```python
from build123d import *

# Parameters (mm, degrees)
SKETCH1_W           = 88.9
SKETCH1_H           = 50.8
BOSS_EXTRUDE1_DEPTH = 114.3
SKETCH2_OUTSIDE_W   = 121.59
SKETCH2_OUTSIDE_H   = 83.49
SKETCH2_OUTSIDE_W_2 = 50.8
SKETCH2_OUTSIDE_H_2 = 50.8
CUT_EXTRUDE1_DEPTH  = 101.6
SKETCH3_R           = 4.9609375
CUT_EXTRUDE2_DEPTH  = 114.769602707
SKETCH4_R           = 5.3578125
CUT_EXTRUDE3_DEPTH  = 41.275
SKETCH5_R           = 2.54
CUT_EXTRUDE4_DEPTH  = 2.54


with BuildPart() as part:
    # Sketch1 → Boss-Extrude1 (new body)
    with BuildSketch(Plane(origin=(0, 0, 0), x_dir=(1, 0, 0), z_dir=(0, 1, 0))):
        Rectangle(SKETCH1_W, SKETCH1_H)
    extrude(amount=BOSS_EXTRUDE1_DEPTH)

    # Sketch2 outside → Cut-Extrude1 (cut)
    with BuildSketch(Plane(origin=(0, 114.3, 0), x_dir=(1, 0, 0), z_dir=(0, 1, 0))):
        Rectangle(SKETCH2_OUTSIDE_W, SKETCH2_OUTSIDE_H)
        Rectangle(SKETCH2_OUTSIDE_W_2, SKETCH2_OUTSIDE_H_2, mode=Mode.SUBTRACT)
    extrude(amount=-CUT_EXTRUDE1_DEPTH, mode=Mode.SUBTRACT)

    # Sketch3 → Cut-Extrude2 (cut, through all)
    with BuildSketch(Plane(origin=(0, 12.7, 0), x_dir=(1, 0, 0), z_dir=(0, 1, 0))):
        with Locations(Location((-34.925, 15.875, 0), (0, 0, 270))):
            Circle(SKETCH3_R)
        with Locations(Location((-34.925, -15.875, 0), (0, 0, 270))):
            Circle(SKETCH3_R)
        with Locations(Location((34.925, -15.875, 0), (0, 0, 270))):
            Circle(SKETCH3_R)
        with Locations(Location((34.925, 15.875, 0), (0, 0, 270))):
            Circle(SKETCH3_R)
    extrude(amount=-CUT_EXTRUDE2_DEPTH, mode=Mode.SUBTRACT)

    # Sketch4 → Cut-Extrude3 (cut)
    with BuildSketch(Plane(origin=(0, 114.3, 0), x_dir=(1, 0, 0), z_dir=(0, 1, 0))):
        with Locations(Location((0, 0, 0), (0, 0, 270))):
            Circle(SKETCH4_R)
    extrude(amount=-CUT_EXTRUDE3_DEPTH, mode=Mode.SUBTRACT)

    # Sketch5 → Cut-Extrude4 (cut)
    with BuildSketch(Plane.XZ):
        with Locations(Location((0, 0, 0), (0, 0, 270))):
            Circle(SKETCH5_R)
    extrude(amount=-CUT_EXTRUDE4_DEPTH, mode=Mode.SUBTRACT)


solid = part.part
```
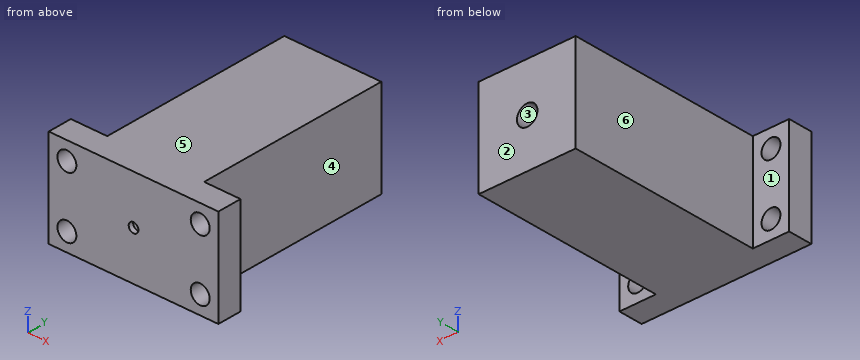
CAD build for the part. Positions are in the model's coordinates, mm. Face numbers are marked on the shaded views. A direction names the side the tool comes from. Round coordinates to 2 decimals unless told otherwise and drop trailing zeros. Write each loop counter-clockwise with the first axis right and the second up, starting at its lowest first coordinate (ties: lowest second). Pieces come first, ordered by that corner, then holes. Notation, with made-up numbers: (67.25, 37.25) - (85.25, 37.25) arc R10 ccw to (85.25, 55.25) - close; hole circle Ø2 at (18, 38.5). An arc over 180 degrees is marked (long way). Return JSON: item names as keys, results as strings. Group by question number.
Item 1: Flat gauge pins, fed straight in: pin 1 Ø8 at (y, z) = (82, -1.5) entering from -X; pin 2 Ø6 at (x, z) = (34.925, 15.875) entering from +Y; pin 3 Ø2.5 at (x, z) = (0.5, 1) entering from -Y; pin 4 Ø9.5 at (x, z) = (31, -9) entering from +Y. Where does each tip first touch, or does it go through?
Item 2: Band-saw the part on D-D on z = 0. List the corners of the cut face in (x, y) (3 decimals), plus the area to 3 significant figures.
Item 3: Band-saw the part on B-B on x = 0. List the corners of the cut face in (y, z) (3 decimals).
Item 4: Mould opens along X. For the marked faces 3, 4, 5 and 6 say: +X half, -X half, draft (parallel to the pull), parting line (faces both ways), or undercut.
Item 5: 3-axis set-ups, long thin cutter, end or side, ignore diameter. For the marked faces 1 and 2: which of +Z, -Z, +X, -X, +Y, -Y reach the whole face in a straight line?
Item 6: Band-saw the part on C-C on x = -32. List the corners of the cut face in (y, z), plus the area to 3 significant figures.
Item 7: Band-saw the part on A-A on z = 19.5. List the corners of the cut face in (x, y).
Item 8: Probe probe 1 along X at (y, z) = (98, 0); probe 2 along X at (y, z) = (7, -19.5); probe 3 along X at (y, z) = (76, 19). List the from-to ranges inside material, lowest first.
Resolved:
{
 "1": {"pin 1": "stops at x = -25.4", "pin 2": "passes through", "pin 3": "stops at y = 2.54", "pin 4": "stops at y = 12.7"},
 "2": {"outline": "(-44.45, 0) - (-2.54, 0) - (-2.54, 2.54) - (2.54, 2.54) - (2.54, 0) - (44.45, 0) - (44.45, 12.7) - (25.4, 12.7) - (25.4, 114.3) - (5.358, 114.3) - (5.358, 73.025) - (-5.358, 73.025) - (-5.358, 114.3) - (-25.4, 114.3) - (-25.4, 12.7) - (-44.45, 12.7) - close", "area": "5,840 mm²"},
 "3": {"outline": "(0, -25.4) - (114.3, -25.4) - (114.3, -5.358) - (73.025, -5.358) - (73.025, 5.358) - (114.3, 5.358) - (114.3, 25.4) - (0, 25.4) - (0, 2.54) - (2.54, 2.54) - (2.54, -2.54) - (0, -2.54) - close"},
 "4": {"face 3": "undercut", "face 4": "+X half", "face 5": "draft", "face 6": "-X half"},
 "5": {"face 1": "+Z, -Z, -X, +Y", "face 2": "+Z, -Z, +X, -X, +Y"},
 "6": {"outline": "(0, -25.4) - (12.7, -25.4) - (12.7, -19.88) - (0, -19.88) - close; (0, -11.87) - (12.7, -11.87) - (12.7, 11.87) - (0, 11.87) - close; (0, 19.88) - (12.7, 19.88) - (12.7, 25.4) - (0, 25.4) - close", "area": "442 mm²"},
 "7": {"outline": "(-44.45, 0) - (-38.31, 0) - (-38.31, 12.7) - (-44.45, 12.7) - close; (-31.54, 0) - (31.54, 0) - (31.54, 12.7) - (25.4, 12.7) - (25.4, 114.3) - (-25.4, 114.3) - (-25.4, 12.7) - (-31.54, 12.7) - close; (38.31, 0) - (44.45, 0) - (44.45, 12.7) - (38.31, 12.7) - close"},
 "8": {"probe 1": "x = -25.4 to -5.36, 5.36 to 25.4", "probe 2": "x = -44.45 to -38.31, -31.54 to 31.54, 38.31 to 44.45", "probe 3": "x = -25.4 to 25.4"}
}
